```python
from build123d import *

# Parameters (mm, degrees)
BOSS_EXTRUDE2_DEPTH         = 25.4
CUT_EXTRUDE2_REACH          = 59.15
SKETCH7_R                   = 7.9375
F_3_8_16_TAPPED_HOLE1_D     = 7.9375
F_3_8_16_TAPPED_HOLE1_DEPTH = 25.4
F_3_8_16_TAPPED_HOLE1_TIP   = 2.384665582


with BuildPart() as part:
    # Sketch1 → Boss-Extrude2 (new body)
    with BuildSketch(Plane(origin=(0, 0, 0), x_dir=(0, 0, -1), z_dir=(1, 0, 0))):
        Polygon((21.525976172, 126.619), (-45.784023828, -19.431), (-45.784023828, -25.781), (30.415976172, -25.781), (30.415976172, 126.619), align=None)
    extrude(amount=BOSS_EXTRUDE2_DEPTH)

    # Sketch4 → CBORE for 3/8 Socket Head Cap Screw1 (revolve, cut)
    with BuildSketch(Plane(origin=(12.7, 96.139, -11.365976172), x_dir=(0, -1, 0), z_dir=(1, 0, 0))):
        Polygon((0, 0), (0, 19.05), (4.9022, 19.05), (4.9022, 9.525), (7.9375, 9.525), (7.9375, 0), align=None)
    revolve(axis=Axis((12.7, 96.139, -5.015976172), (0, 0, -1)), mode=Mode.SUBTRACT)

    # Sketch6 → CBORE for 3/8 Socket Head Cap Screw2 (revolve, cut)
    with BuildSketch(Plane(origin=(12.7, 37.719, -10.095976172), x_dir=(0, -1, 0), z_dir=(1, 0, 0))):
        Polygon((0, 0), (0, 20.32), (4.9022, 20.32), (4.9022, 9.525), (7.9375, 9.525), (7.9375, 0), align=None)
    revolve(axis=Axis((12.7, 37.719, -3.745976172), (0, 0, -1)), mode=Mode.SUBTRACT)

    # Sketch7 → Cut-Extrude2 (cut, up to next)
    with BuildSketch(Plane(origin=(0, 96.139, -11.365976172), x_dir=(1, 0, 0), z_dir=(0, 0, 1)), mode=Mode.PRIVATE) as cut_extrude2_sk1:
        with Locations((12.7, -58.42)):
            Circle(SKETCH7_R)
    cut_extrude2_tool1 = extrude(cut_extrude2_sk1.sketch, amount=CUT_EXTRUDE2_REACH, mode=Mode.PRIVATE) & part.part
    add(cut_extrude2_tool1.solids().sort_by_distance((12.7, 37.719, -11.365976))[0], mode=Mode.SUBTRACT)
    # Sketch7 → Cut-Extrude2 (cut, up to next)
    with BuildSketch(Plane(origin=(0, 96.139, -11.365976172), x_dir=(1, 0, 0), z_dir=(0, 0, 1)), mode=Mode.PRIVATE) as cut_extrude2_sk2:
        with Locations((12.7, 0)):
            Circle(SKETCH7_R)
    cut_extrude2_tool2 = extrude(cut_extrude2_sk2.sketch, amount=CUT_EXTRUDE2_REACH, mode=Mode.PRIVATE) & part.part
    add(cut_extrude2_tool2.solids().sort_by_distance((12.7, 96.139, -11.365976))[0], mode=Mode.SUBTRACT)

    # 3/8-16 Tapped Hole1
    with Locations(Plane(origin=(12.7, -25.781, -15.175976172), x_dir=(0, 0, -1), z_dir=(0, -1, 0))):
        with Locations((0, 0), (-40.64, 0)):
            Hole(F_3_8_16_TAPPED_HOLE1_D / 2, depth=F_3_8_16_TAPPED_HOLE1_DEPTH)
            with Locations((0, 0, -(F_3_8_16_TAPPED_HOLE1_DEPTH + F_3_8_16_TAPPED_HOLE1_TIP / 2))):  # 118° drill point
                Cone(0, F_3_8_16_TAPPED_HOLE1_D / 2, F_3_8_16_TAPPED_HOLE1_TIP, mode=Mode.SUBTRACT)


solid = part.part
```
Design review of the part built by this model. Coordinates are the model's own, in mm. A direction names the side the tool comes from. Coordinates: 2 decimals unless noted, no trailing zeros. Order: outer loops, then holes, each group sorted by start corner. A loop starts at its lowest first (then second) coordinate and runs counter-clockwise, first axis right, second up. Notation, with made-up numbers: (56, 13.5) -> (84, 13.5) arc R17 ccw to (84, 42.5) -> close; hole circle Ø6 at (83, 17.25). An arc over 180 degrees is marked (long way). One line per item, written item: value. Start each with the question number.
Q1. Take a section at D-D, the plane z = 15. State the section outline as (x, y) points (1 decimal), then the cut area to 3 significant figures.
Q2. Take a section at B-B, the plane x = 10.5. Give the number of separate pieces and of enclosed holes in the cut face, then the cut area to 3 significant figures.
Q3. For probe 1 along Y at (x, z) = (12.7, -26.25); probe 2 along Z at (x, y) = (12.7, -20); probe 3 along Y at (x, z) = (8.5, -17), list the stretches that pass through material, from the lowest coordinate up.
Q4. Take a section at C-C, the plane y = 112. State the section outline as (x, z) points.
Q5. Insertion check: pin 1 Ø5 at (x, y) = (16, 38.5) entering from +Z; pin 2 Ø3 at (x, z) = (13, 16) entering from +Y; pin 3 Ø9 at (x, z) = (12.7, -15.18) entering from +Y. Each pin has a flat end and moves straight along its axis. Give the tip position at first contact, or say it passes through.
Q6. Tool access review of faces 4 (the flat face through (13, 43, -19.621)), 5 (the cylindrical face through (10.29, -12.9, 22.31)), 6 (the flat face through (13, 126.619, -26)): name each direction out of +Z, -Z, +X, -X, +Y, -Y from which nothing blocks a thin tool from reaching the whole face with its end or side.
Q7. Mouldability with a two-part tool opening along Z and no side actions: class faces 1 (the flat face through (12.522, 54.616, 11.658)), 2 (the cylindrical face through (12.484, 101.036, -25.587)), 3 (the conical face through (12.3, 1.6, 26)) as pulls with the +Z half, pulls with the -Z half, needs draft (parallel to the pull), parting line crosses it, or undercut.
Q8. Take a section at A-A, the plane z = 3. State the section outline as (x, y) points (1 decimal).
Values follow:
1. outline: (0, -25.8) -> (25.4, -25.8) -> (25.4, 47.4) -> (0, 47.4) -> close; hole circle Ø15.9 at (12.7, 37.7)
1. area: 1,660 mm2
2. separate pieces: 3
2. enclosed holes: 0
2. area: 5,370 mm2
3. probe 1: y = -25.78 to 32.82, 42.62 to 91.24, 101.04 to 126.62
3. probe 2: z = -30.42 to -19.14, -11.21 to 21.5, 29.43 to 45.78
3. probe 3: y = -25.78 to 30.98, 44.45 to 89.4, 102.87 to 116.8
4. outline: (0, -30.42) -> (25.4, -30.42) -> (25.4, -14.79) -> (0, -14.79) -> close
5. pin 1: stops at z = -19.62
5. pin 2: stops at y = 48.45
5. pin 3: stops at y = 122.61
6. face 4: +Z
6. face 5: -Y
6. face 6: +Z, -Z, +X, -X, +Y
7. face 1: pulls with the +Z half
7. face 2: needs draft
7. face 3: undercut
8. outline: (0, -25.8) -> (25.4, -25.8) -> (25.4, 73.4) -> (0, 73.4) -> close; hole circle Ø15.9 at (12.7, 37.7)
